The drawing under review shows one solid part. Ordinate dimensions are in mm from its lowest x, y, z. A direction names the side the tool comes from. Round coordinates to 2 decimals unless told otherwise and drop trailing zeros. Order: outer loops, then holes, each group sorted by start corner. A loop starts at its lowest first (then second) coordinate and runs counter-clockwise, first axis right, second up. Notation, with made-up numbers: M -14,-6 L 3,-6 A14 ccw 3,17 Z; hole C -14,23.25 d11. An arc over 180 degrees is marked long. Use a Markdown table: item, result.
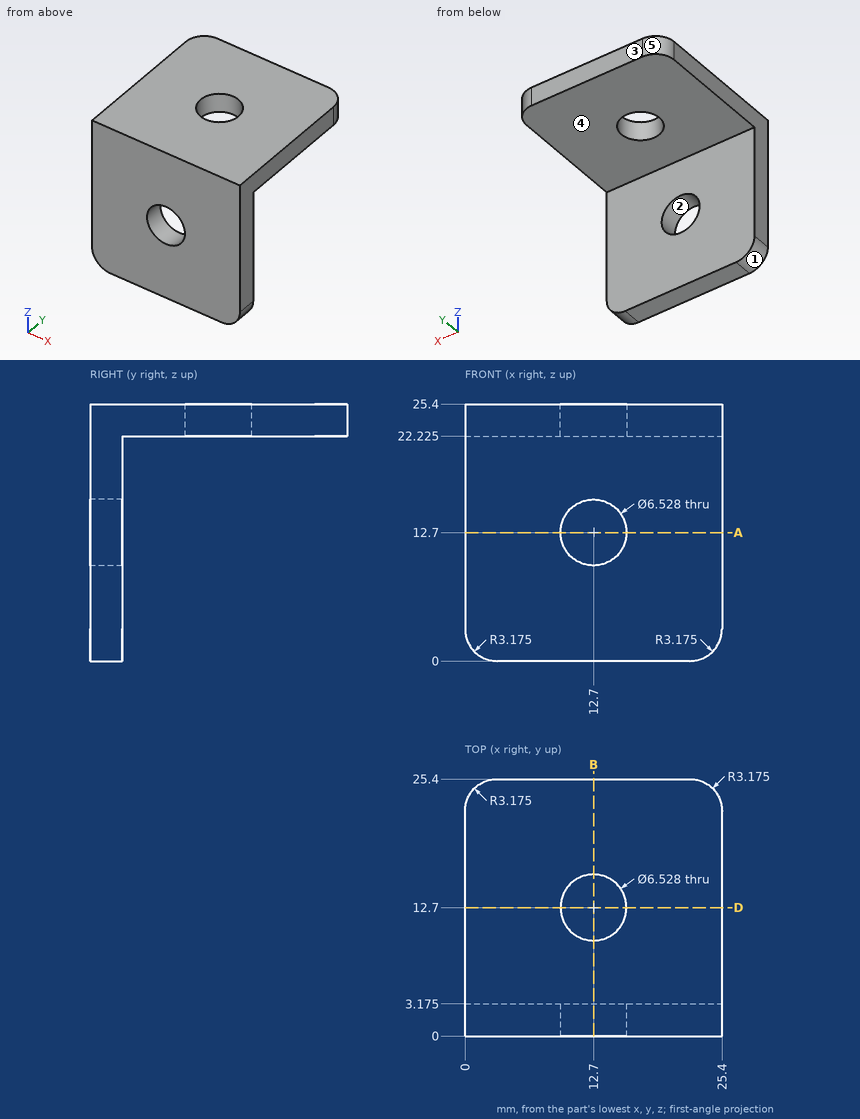
Q1. Clearance check with flat-ended pins moving along their axes: pin 1 (4 mm diameter, centred on x = 16, y = 22.5, fed in from -Z) (3 decimals); pin 2 (11 mm diameter, centred on x = 16, z = 11.5, fed in from +Y) (3 decimals). State where each tip first meets the part, or that it passes through.
Determined:
| item | result |
|---|---|
| pin 1 | stops at z = 22.225 |
| pin 2 | stops at y = 3.175 |
Q2. Wall thickness on line 1 along Z through (x, y) = (3.5, 11.5) (3 decimals); line 2 along Y through (x, z) = (17, 18) (3 decimals); line 3 along X through (y, z) = (13.75, 24.5): over which ranges is each line inside the solid? List them lowest first. Write a range as [from, to].
Determined:
| item | result |
|---|---|
| line 1 | z = [22.225, 25.4] |
| line 2 | y = [0, 3.175] |
| line 3 | x = [0, 9.61], [15.79, 25.4] |
Q3. Add section D-D (y = 12.7). Write out the cut boundary in (x, z) (1 decimal).
Determined:
| item | result |
|---|---|
| outline | M 0,22.2 L 9.4,22.2 L 9.4,25.4 L 0,25.4 Z; M 16,22.2 L 25.4,22.2 L 25.4,25.4 L 16,25.4 Z |
Q4. Machinability: for the marked faces 4 and 5, which of the approach directions +Z, -Z, +X, -X, +Y, -Y give a long, thin tool a straight path to every point of the face, cutting with its end or side? Answer none if there is none.
Determined:
| item | result |
|---|---|
| face 4 | -Z, +X, -X, +Y |
| face 5 | +Z, -Z, -X, +Y |
Q5. Add section A-A (z = 12.7). Write out the cut boundary in (x, y) (1 decimal), then the cut area to 3 significant figures.
Determined:
| item | result |
|---|---|
| outline | M 0,0 L 9.4,0 L 9.4,3.2 L 0,3.2 Z; M 16,0 L 25.4,0 L 25.4,3.2 L 16,3.2 Z |
| area | 59.9 mm^2 |
Q6. Add section B-B (x = 12.7). Write out the cut boundary in (y, z) (1 decimal), then the cut area to 3 significant figures.
Determined:
| item | result |
|---|---|
| outline | M 0,0 L 3.2,0 L 3.2,9.4 L 0,9.4 Z; M 0,16 L 3.2,16 L 3.2,22.2 L 9.4,22.2 L 9.4,25.4 L 0,25.4 Z; M 16,22.2 L 25.4,22.2 L 25.4,25.4 L 16,25.4 Z |
| area | 110 mm^2 |
Q7. Draft analysis for pull direction X (two halves, no side actions). For the marked faces 1, 2 and 3, state which applies: pulls with the +X half, pulls with the -X half, needs draft (parallel to the pull), parting line crosses it, or undercut.
Determined:
| item | result |
|---|---|
| face 1 | pulls with the -X half |
| face 2 | undercut |
| face 3 | needs draft |
